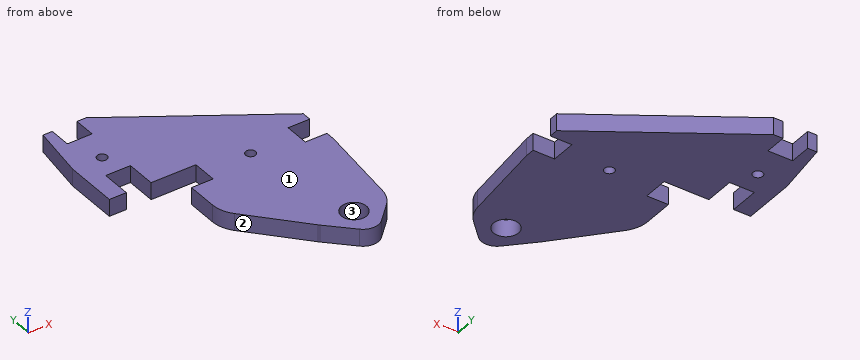
from build123d import *

# Parameters (mm, degrees)
F0_R     = 4.05
F0_R_2   = 1.6
F1_DEPTH = 5.5


with BuildPart() as f1:
    # F0 (on Top) → F1 (new body)
    with BuildSketch(Plane.XY):
        with BuildLine():
            Line((-22.2, 41.5), (-22.2, 37.5))
            Line((-22.2, 37.5), (-22.2, 33.5))
            Line((-22.2, 33.5), (-29.2, 33.5))
            Line((-29.2, 33.5), (-29.2, 23.829429))
            ThreePointArc((-29.2, 23.829429), (-28.538679, 20.253248), (-26.642186, 17.150068))
            Line((-26.642186, 17.150068), (-11.430273, 0.200861))
            ThreePointArc((-11.430273, 0.200861), (-11.247357, 0.002505), (-11.059155, -0.190845))
            Line((-11.059155, -0.190845), (-3.535534, -7.714466))
            ThreePointArc((-3.535534, -7.714466), (0, -9.178932), (3.535534, -7.714466))
            Line((3.535534, -7.714466), (8.764601, -2.485399))
            ThreePointArc((8.764601, -2.485399), (10.709292, 0.259459), (11.633753, 3.493874))
            Line((11.633753, 3.493874), (14.6, 30.5))
            Line((14.6, 30.5), (14.6, 33.5))
            Line((14.6, 33.5), (7.6, 33.5))
            Line((7.6, 33.5), (7.6, 37.5))
            Line((7.6, 37.5), (7.6, 41.5))
            Line((7.6, 41.5), (14.6, 41.5))
            Line((14.6, 41.5), (14.6, 44.5))
            Line((14.6, 44.5), (-33.7, 75.9))
            Line((-33.7, 75.9), (-36.7, 75.9))
            Line((-36.7, 75.9), (-36.7, 68.9))
            Line((-36.7, 68.9), (-40.7, 68.9))
            Line((-40.7, 68.9), (-44.7, 68.9))
            Line((-44.7, 68.9), (-44.7, 75.9))
            Line((-44.7, 75.9), (-47.7, 75.9))
            Line((-47.7, 75.9), (-50.2, 58.5))
            Line((-50.2, 58.5), (-50.2, 41.5))
            Line((-50.2, 41.5), (-44.7, 41.5))
            Line((-44.7, 41.5), (-44.7, 51.1))
            Line((-44.7, 51.1), (-40.7, 51.1))
            Line((-40.7, 51.1), (-36.7, 51.1))
            Line((-36.7, 51.1), (-36.7, 41.5))
            Line((-36.7, 41.5), (-22.2, 41.5))
        make_face()
        Circle(F0_R, mode=Mode.SUBTRACT)
        with Locations((-40.7, 58.5)):
            Circle(F0_R_2, mode=Mode.SUBTRACT)
        with Locations((-7.3, 37.5)):
            Circle(F0_R_2, mode=Mode.SUBTRACT)
    extrude(amount=F1_DEPTH)


solid = f1.part
Can you work these out from the model? Positions are in its coordinate system, mm. Face numbers are marked on the shaded views. Round coordinates to 2 decimals unless told otherwise and drop trailing zeros. Order: outer loops, then holes, each group sorted by start corner. A loop starts at its lowest first (then second) coordinate and runs counter-clockwise, first axis right, second up. Notation, with made-up numbers: M 83,15 L 94,15 A19 ccw 94,25 Z; hole C 15,48.25 d1. An arc over 180 degrees is marked long. Use a Markdown table: item, result.
1) Imagine slicing it at B-B (y = 37.5). List the corners of the cut face in (x, z) for me, then the cut area to 3 significant figures.
Geometry says:
| item | result |
|---|---|
| outline | M -22.2,0 L -8.9,0 L -8.9,5.5 L -22.2,5.5 Z; M -5.7,0 L 7.6,0 L 7.6,5.5 L -5.7,5.5 Z |
| area | 146 mm² |
2) Imagine slicing it at A-A (x = -40.7). List the corners of the cut face in (y, z) for me, then the cut area to 3 significant figures.
Geometry says:
| item | result |
|---|---|
| outline | M 51.1,0 L 56.9,0 L 56.9,5.5 L 51.1,5.5 Z; M 60.1,0 L 68.9,0 L 68.9,5.5 L 60.1,5.5 Z |
| area | 80.3 mm² |
3) I'm going to push flat-ended pins straight in: P1, Ø3, axis at x = -7.3, y = 37.5, coming from the +Z side; P2, Ø3, axis at x = -7.5, z = 4.5, coming from the -Y side; P3, Ø3, axis at y = 29.5, z = 2, coming from the -X side; P4, Ø1, axis at y = 28, z = 3.5, coming from the +X side. Where does each tip first touch, or does it pass through?
Geometry says:
| item | result |
|---|---|
| P1 | passes through |
| P2 | stops at y = -5.25 |
| P3 | stops at x = -29.2 |
| P4 | stops at x = 14.38 |
4) Imagine slicing it at C-C (z = 2.65). Give the number of separate pieces and of enclosed holes in the cut face, then the cut area to 3 significant figures.
Geometry says:
| item | result |
|---|---|
| separate pieces | 1 |
| enclosed holes | 3 |
| area | 2,840 mm² |
5) Imagine slicing it at D-D (x = -20.5). List the corners of the cut face in (y, z) for me, then the cut area to 3 significant figures.
Geometry says:
| item | result |
|---|---|
| outline | M 10.31,0 L 67.32,0 L 67.32,5.5 L 10.31,5.5 Z |
| area | 314 mm² |
6) If we mould it in two halves opening along Y, with no side actions, what happens to the marked faces 1, 2 and 3? For each: +Y half, -Y half, draft (parallel to the pull), parting line (faces both ways), or undercut.
Geometry says:
| item | result |
|---|---|
| face 1 | draft |
| face 2 | -Y half |
| face 3 | undercut |
7) If I drill on line 1 along Y through (x, z) = (-40.7, 2.4); line 2 along Y through (x, z) = (-27, 0.7); line 3 along Y through (x, z) = (-36, 1), over which ranges is the centre line in solid material (lowest first)?
Geometry says:
| item | result |
|---|---|
| line 1 | y = 51.1 to 56.9, 60.1 to 68.9 |
| line 2 | y = 17.57 to 33.5, 41.5 to 71.54 |
| line 3 | y = 41.5 to 75.9 |
